```python
from build123d import *

# Parameters (mm, degrees)
PAD_DEPTH     = 70
PAD001_DEPTH  = 200
PAD002_DEPTH  = 70
SKETCH003_R   = 2.5
PAD003_DEPTH  = 5
SKETCH004_R   = 8.5
SKETCH004_R_2 = 2.5
PAD004_DEPTH  = 205


with BuildPart() as part:
    # Sketch → Pad (new body)
    with BuildSketch(Plane.XY):
        with BuildLine():
            ThreePointArc((-29.848016, -3.015947), (29.920505, -2.182515), (-29.094406, 7.315431))
            ThreePointArc((-29.094406, 7.315431), (-29.072912, 3.034578), (-26.991574, -0.706304))
            Line((-26.991574, -0.706304), (-12.739759, -15.728805))
            ThreePointArc((-12.739759, -15.728805), (-11.4789, -15.911046), (-11.008743, -14.727014))
            Line((-11.008743, -14.727014), (-18.604437, 10.709188))
            ThreePointArc((-18.160969, 13.282665), (-18.684551, 12.047942), (-18.604437, 10.709188))
            ThreePointArc((-20.499669, -9.27435), (22.380035, -2.320351), (-18.160969, 13.282665))
            ThreePointArc((-20.499669, -9.27435), (-21.232479, -7.959372), (-22.173804, -6.784601))
            Line((-22.173804, -6.784601), (-26.991574, -1.706304))
            ThreePointArc((-26.991574, -1.706304), (-28.888073, -1.339771), (-29.848016, -3.015947))
        make_face()
    extrude(amount=PAD_DEPTH)

    # Sketch001 → Pad001 (join)
    with BuildSketch(Plane.XY):
        Polygon((23.5, -48.619546), (11.75, -28.267949), (-11.75, -28.267949), (-23.5, -48.619546), (-11.75, -68.971143), (11.75, -68.971143), align=None)
        Polygon((21.5, -48.619546), (10.75, -30), (-10.75, -30), (-21.5, -48.619546), (-10.75, -67.239092), (10.75, -67.239092), align=None, mode=Mode.SUBTRACT)
    extrude(amount=PAD001_DEPTH)

    # Sketch002 → Pad002 (join)
    with BuildSketch(Plane.XY):
        Polygon((-18.915001, -22.616726), (-23.5, -48.619546), (-11.75, -28.267949), (-6.937376, -28.267949), align=None)
        Polygon((23.5, -48.619546), (19.018119, -23.201534), (10.046046, -28.267949), (11.75, -28.267949), align=None)
    extrude(amount=PAD002_DEPTH)

    # Sketch003 → Pad003 (join)
    with BuildSketch(Plane.XY):
        Polygon((21.5, -48.619546), (10.75, -30), (-10.75, -30), (-21.5, -48.619546), (-10.75, -67.239092), (10.75, -67.239092), align=None)
        with Locations((0, -48.619546)):
            Circle(SKETCH003_R, mode=Mode.SUBTRACT)
    extrude(amount=PAD003_DEPTH)

    # Sketch004 → Pad004 (join)
    with BuildSketch(Plane.XY):
        with Locations((0, -48.619546)):
            Circle(SKETCH004_R)
        with Locations((0, -48.619546)):
            Circle(SKETCH004_R_2, mode=Mode.SUBTRACT)
    extrude(amount=PAD004_DEPTH)


solid = part.part
```
Part model, mm, in its own coordinate system. A direction names the side the tool comes from. Coordinates: 2 decimals unless noted, no trailing zeros. Order: outer loops, then holes, each group sorted by start corner. A loop starts at its lowest first (then second) coordinate and runs counter-clockwise, first axis right, second up. Notation, with made-up numbers: (61.25, 77.5) - (97.25, 77.5) arc R18 cw to (97.25, 84.5) - close; hole circle Ø1 at (60.25, 56). An arc over 180 degrees is marked (long way). Return JSON: item names as keys, results as strings. Group by question number.
Item 1: Cut at C-C (x = 15). List the corners of the cut face in (y, z), plus the area to 3 significant figures.
Item 2: Cut at B-B (z = 60.5). State how many separate pieces and enclosed holes the cut face has, plus the area to 3 significant figures.
Item 3: Pin check, flat tips, straight feed: pin 1 (10 mm diameter, centred on x = 17.5, y = -27.5, fed in from +Z); pin 2 (17 mm diameter, centred on x = 0.5, z = 125, fed in from +Y); pin 3 (8 mm diameter, centred on y = -31, z = 170, fed in from -X). Stop position of each tip, or through.
Item 4: Drill centre lines: probe 1 along Y at (x, z) = (0, 128.5); probe 2 along Y at (x, z) = (0, 51); probe 3 along X at (y, z) = (-15, 61). Where is each one in solid material? Low to high. Write a range as from..to.
Item 5: Cut at A-A (z = 171.5). List the corners of the cut face in (x, y), plus the area to 3 significant figures.
Item 6: Which spindle directions (+Z, -Z, +X, -X, +Y, -Y) get a long thin tool onto all of the face, cutting with end or side? Do faces 5 (the face through (-16.2, -57.8, 101.1)), 6 (the face through (0, -28.268, 134)), 7 (the face through (-26.51, -14.04, 34.51)), 8 (the face through (21.29, -36.09, 34.51)). Say none if no direction does.
Item 7: Pull direction X, two halves, no side cores. Call faces 1 (the face through (0, -30, 101)), 2 (the face through (-21.228, -35.733, 34.51)), 3 (the face through (1.34, -46.51, 101.06)), 4 (the face through (0, -30, 0)): pulls with the +X half, pulls with the -X half, needs draft (parallel to the pull), parting line crosses it, or undercut.
Check values:
{
 "1": {"outline": "(-63.34, 0) - (-16.77, 0) - (-16.77, 70) - (-33.9, 70) - (-33.9, 200) - (-37.36, 200) - (-37.36, 5) - (-59.88, 5) - (-59.88, 200) - (-63.34, 200) - close; (16.77, 0) - (25.98, 0) - (25.98, 70) - (16.77, 70) - close", "area": "3,340 mm2"},
 "2": {"separate pieces": "2", "enclosed holes": "2", "area": "2,000 mm2"},
 "3": {"pin 1": "stops at z = 70", "pin 2": "stops at y = -28.27", "pin 3": "stops at x = -15.64"},
 "4": {"probe 1": "y = -68.97..-67.24, -57.12..-51.12, -46.12..-40.12, -30..-28.27", "probe 2": "y = -68.97..-67.24, -57.12..-51.12, -46.12..-40.12, -30..-22.5, 22.5..30", "probe 3": "x = -25.98..-16.77, -13.43..-10.97, 16.77..25.98"},
 "5": {"outline": "(-23.5, -48.62) - (-11.75, -68.97) - (11.75, -68.97) - (23.5, -48.62) - (11.75, -28.27) - (-11.75, -28.27) - close; circle Ø17 at (0, -48.62); hole (-21.5, -48.62) - (-10.75, -67.24) - (10.75, -67.24) - (21.5, -48.62) - (10.75, -30) - (-10.75, -30) - close; hole circle Ø5 at (0, -48.62)", "area": "441 mm2"},
 "6": {"face 5": "+Z", "face 6": "+Z, +X, -X, +Y", "face 7": "+Z, -Z, -X", "face 8": "+Z, -Z, +X"},
 "7": {"face 1": "undercut", "face 2": "pulls with the -X half", "face 3": "undercut", "face 4": "needs draft"}
}
